Could you check a few things on this model? Use its own coordinates, in mm. A direction names the side the tool comes from. Round coordinates to 2 decimals unless told otherwise and drop trailing zeros. Write each loop counter-clockwise with the first axis right and the second up, starting at its lowest first coordinate (ties: lowest second). Pieces come first, ordered by that corner, then holes. Notation, with made-up numbers: (-10.5, 54) -> (3.5, 54) arc R28 cw to (3.5, 75) -> close; hole circle Ø1 at (30, -40). An arc over 180 degrees is marked (long way). Answer in a Markdown table with one row per item.
from build123d import *

# Parameters (mm, degrees)
F0_W     = 50
F0_H     = 20
F1_DEPTH = 30
F2_W     = 14
F2_H     = 20
F3_DEPTH = 20
F4_R     = 5
F5_DEPTH = 10
F6_R     = 2.5
F7_DEPTH = 25


with BuildPart() as f1:
    # F0 (on Front) → F1 (new body)
    with BuildSketch(Plane.XZ):
        Rectangle(F0_W, F0_H)
    extrude(amount=F1_DEPTH)

    # F2 (on face) → F3 (cut)
    with BuildSketch(Plane.XZ.offset(30)):
        with Locations((-18, 0)):
            Rectangle(F2_W, F2_H)
        with Locations((18, 0)):
            Rectangle(F2_W, F2_H)
    extrude(amount=-F3_DEPTH, mode=Mode.SUBTRACT)

    # F4 (on face) → F5 (cut)
    with BuildSketch(Plane.XY.offset(10)):
        with Locations((0, -22)):
            Circle(F4_R)
    extrude(amount=-F5_DEPTH, mode=Mode.SUBTRACT)

    # F6 (on face) → F7 (cut)
    with BuildSketch(Plane.XZ.offset(10)):
        with Locations((-19, 0)):
            Circle(F6_R)
        with Locations((19, 0)):
            Circle(F6_R)
    extrude(amount=-F7_DEPTH, mode=Mode.SUBTRACT)


solid = f1.part
1) Thinking about a two-plate mould opening in Y: for faces 5 (the face through (0, 0, 0)), 6 (the face through (0, -30, 0)), 7 (the face through (11, -20, 0)), 8 (the face through (-1.08, -26.88, 5.07)), which applies, +Y half, -Y half, draft (parallel to the pull), parting line (faces both ways), or undercut?
Findings:
| item | result |
|---|---|
| face 5 | +Y half |
| face 6 | -Y half |
| face 7 | draft |
| face 8 | undercut |
2) Imagine slicing it at B-B, the plane y = -18. Please give me the cut outline in (x, z), plus the area to 3 significant figures.
Findings:
| item | result |
|---|---|
| outline | (-11, -10) -> (11, -10) -> (11, 10) -> (3, 10) -> (3, 0) -> (-3, 0) -> (-3, 10) -> (-11, 10) -> close |
| area | 380 mm^2 |
3) For pin 1 (4 mm diameter, centred on y = -17.5, z = -8, fed in from -X); pin 2 (3 mm diameter, centred on y = -21.5, z = -6.5, fed in from +X); pin 3 (6.5 mm diameter, centred on x = 19, z = 0, fed in from -Y), each with a flat end and sliding along its axis, tell me the tip position at first contact or that it passes through.
Findings:
| item | result |
|---|---|
| pin 1 | stops at x = -11 |
| pin 2 | stops at x = 11 |
| pin 3 | stops at y = -10 |
4) Imagine slicing it at C-C, the plane y = -8.75. Please give me the cut outline in (x, z), plus the area to 3 significant figures.
Findings:
| item | result |
|---|---|
| outline | (-25, -10) -> (25, -10) -> (25, 10) -> (-25, 10) -> close; hole circle Ø5 at (-19, 0); hole circle Ø5 at (19, 0) |
| area | 961 mm^2 |
5) Imagine slicing it at D-D, the plane x = 0. Please give me the cut outline in (y, z).
Findings:
| item | result |
|---|---|
| outline | (-30, -10) -> (0, -10) -> (0, 10) -> (-17, 10) -> (-17, 0) -> (-27, 0) -> (-27, 10) -> (-30, 10) -> close |
6) Imagine slicing it at A-A, the plane x = -19. Please give me the cut outline in (y, z).
Findings:
| item | result |
|---|---|
| outline | (-10, -10) -> (0, -10) -> (0, -2.5) -> (-10, -2.5) -> close; (-10, 2.5) -> (0, 2.5) -> (0, 10) -> (-10, 10) -> close |
7) Please list where these lines run through material, in increasing order: line 1 (Z direction, x = 19, y = -6); line 2 (Y direction, x = 0, z = 8); line 3 (Y direction, x = 12.5, z = 7.75).
Findings:
| item | result |
|---|---|
| line 1 | z = -10 to -2.5, 2.5 to 10 |
| line 2 | y = -30 to -27, -17 to 0 |
| line 3 | y = -10 to 0 |
8) For faces 1 (the face through (-17, -10, 2)), 2 (the face through (16, -10, 0)), 3 (the face through (0, -11, -10)), 4 (the face through (0, -22, 0)), which set-ups out of +Z, -Z, +X, -X, +Y, -Y let a thin tool reach every point of the face, with its end or its side?
Findings:
| item | result |
|---|---|
| face 1 | +Z, -Z, -X, -Y |
| face 2 | +Z, -Z, +X, -Y |
| face 3 | -Z, +X, -X, +Y, -Y |
| face 4 | +Z |
